from build123d import *

# Parameters (mm, degrees)
SKETCH1_W           = 25.4
SKETCH1_H           = 25.4
SKETCH1_W_2         = 19.05
SKETCH1_H_2         = 19.05
BOSS_EXTRUDE1_DEPTH = 685.8
SKETCH3_W           = 25.4
SKETCH3_H           = 26.296014982
CUT_EXTRUDE2_DEPTH  = 663.667216417


with BuildPart() as part:
    # Sketch1 → Boss-Extrude1 (new body)
    with BuildSketch(Plane.XY):
        Rectangle(SKETCH1_W, SKETCH1_H)
        Rectangle(SKETCH1_W_2, SKETCH1_H_2, mode=Mode.SUBTRACT)
    extrude(amount=BOSS_EXTRUDE1_DEPTH)

    # Sketch3 → Cut-Extrude2 (cut, through all)
    with BuildSketch(Plane(origin=(0, -170.599261314, 636.685110958), x_dir=(-1, 0, 0), z_dir=(0, -0.25881904510250786, 0.9659258262890718))):
        with Locations((0, -176.617351634)):
            Rectangle(SKETCH3_W, SKETCH3_H)
    extrude(amount=CUT_EXTRUDE2_DEPTH, mode=Mode.SUBTRACT)


solid = part.part
The model under review builds one solid part; all positions refer to its coordinate system, in mm. A direction names the side the tool comes from. Give positions to 0.01 mm unless a question says otherwise; leave off trailing zeros. Write each loop counter-clockwise with the first axis right and the second up, starting at its lowest first coordinate (ties: lowest second). Pieces come first, ordered by that corner, then holes. Notation, with made-up numbers: M 21.5,79 L 68.5,79 A4 cw 68.5,85 Z; hole C 15,22 d6. An arc over 180 degrees is marked long. One line per question, with ' | ' between items. Start each with the question number.
Item 1: We need section B-B on y = -2.25. Write out the cut boundary in (x, z) (3 decimals), plus the area to 3 significant figures.
Item 2: We need section C-C on z = 63. Write out the cut boundary in (x, y) (3 decimals), plus the area to 3 significant figures.
Item 3: Wall thickness on line 1 (X direction, y = -6, z = 226) (3 decimals); line 2 (Z direction, x = -7.75, y = -10.5): over which ranges is each line inside the solid? List them lowest first. Write a range as from..to.
Item 4: Draft analysis for pull direction X (two halves, no side actions). For faces 3 (the flat face through (0, 12.7, 338)), 4 (the flat face through (9.525, 0, 338)), 5 (the flat face through (-12.7, 0, 338)), state which applies: released by +X, released by -X, zero draft, split by the parting line, or undercut.
Item 5: For pin 1 (10 mm diameter, centred on x = 7.5, y = 9.5, fed in from +Z), flat-tipped, find the tip position at first contact; note if it passes through.
Item 6: We need section A-A on x = -3.5. Write out the cut boundary in (y, z) (3 decimals).
Item 7: For faces 1 (the flat face through (-11.11, -0.18, 682.35)), 2 (the flat face through (0, 9.525, 338)), list the 3-axis set-ups (+Z, -Z, +X, -X, +Y, -Y) from which the entire face can be reached by the end or side of a thin tool; tool diameter is ignored.
Results found:
1) outline: M -12.7,0 L -9.525,0 L -9.525,681.794 L -12.7,681.794 Z; M 9.525,0 L 12.7,0 L 12.7,681.794 L 9.525,681.794 Z | area: 4,330 mm2
2) outline: M -12.7,-12.7 L 12.7,-12.7 L 12.7,12.7 L -12.7,12.7 Z; hole M -9.525,-9.525 L 9.525,-9.525 L 9.525,9.525 L -9.525,9.525 Z | area: 282 mm2
3) line 1: x = -12.7..-9.525, 9.525..12.7 | line 2: z = 0..679.58
4) face 3: zero draft | face 4: undercut | face 5: released by -X
5) pin 1: stops at z = 685.8
6) outline: M -12.7,0 L -9.525,0 L -9.525,679.845 L -12.7,678.994 Z; M 9.525,0 L 12.7,0 L 12.7,685.8 L 9.525,684.949 Z
7) face 1: +Z, +X, -X, -Y | face 2: +Z, -Z
